```python
from build123d import *

# Parameters (mm, degrees)
F1_DEPTH = 3
F0_W     = 185
F0_H     = 265
F2_DEPTH = 74.8
F3_R     = 6.75
F4_R     = 2.99999


# Not quite as in the source:
# - a fillet or chamfer is up to 0.001 mm smaller than in the source, because OpenCascade refuses the exact size
# - ends of sketch curves that miss each other by under 0.0002 mm in the source are joined


with BuildPart() as f1:
    # F0 (on Top) → F1 (new body)
    with BuildSketch(Plane.XY):
        with BuildLine():
            Line((70.6, 125.95), (70.6, 129))
            Line((70.6, 129), (-70.6, 129))
            Line((-70.6, 129), (-70.6, 125.95))
            ThreePointArc((-70.6, 125.95), (-72.577029227, 121.177029227), (-77.35, 119.2))
            Line((-77.35, 119.2), (-89, 119.2))
            Line((-89, 119.2), (-89, 6.080118008))
            Line((-89, 6.080118008), (-86, 6.080118008))
            ThreePointArc((-86, 6.080118008), (-79.25, -0.669881992), (-86, -7.419881992))
            Line((-86, -7.419881992), (-89, -7.419881992))
            Line((-89, -7.419881992), (-89, -119.2))
            Line((-89, -119.2), (-77.3450501441, -119.2))
            ThreePointArc((-77.3450501441, -119.2), (-72.4815603684, -121.2692984284), (-70.6, -126.2084541623))
            Line((-70.6, -126.2084541623), (-70.6, -129))
            Line((-70.6, -129), (70.6, -129))
            Line((70.6, -129), (70.6, -125.95))
            ThreePointArc((70.6, -125.95), (72.577029227, -121.177029227), (77.35, -119.2))
            Line((77.35, -119.2), (89, -119.2))
            Line((89, -119.2), (89, -6.75))
            Line((89, -6.75), (86, -6.75))
            ThreePointArc((86, -6.75), (79.25, 0), (86, 6.75))
            Line((86, 6.75), (89, 6.75))
            Line((89, 6.75), (89, 119.2))
            Line((89, 119.2), (77.35, 119.2))
            ThreePointArc((77.35, 119.2), (72.577029227, 121.177029227), (70.6, 125.95))
        make_face()
    extrude(amount=F1_DEPTH)

    # F0 (on Top) → F2 (join)
    with BuildSketch(Plane.XY):
        Rectangle(F0_W, F0_H)
        Polygon((70.6, 129), (89, 129), (89, 119.2), (89, 6.75), (89, -6.75), (89, -119.2), (89, -129), (70.6, -129), (-70.6, -129), (-89, -129), (-89, -119.2), (-89, -7.419881992), (-89, 6.080118008), (-89, 119.2), (-89, 129), (-70.6, 129), align=None, mode=Mode.SUBTRACT)
        with BuildLine():
            Line((-77.3450501441, -119.2), (-89, -119.2))
            Line((-89, -119.2), (-89, -129))
            Line((-89, -129), (-70.6, -129))
            Line((-70.6, -129), (-70.6, -126.2084541623))
            ThreePointArc((-70.6, -126.2084541623), (-72.4815603684, -121.2692984284), (-77.3450501441, -119.2))
        make_face()
        with BuildLine():
            Line((89, -129), (89, -119.2))
            Line((89, -119.2), (77.35, -119.2))
            ThreePointArc((77.35, -119.2), (72.577029227, -121.177029227), (70.6, -125.95))
            Line((70.6, -125.95), (70.6, -129.000006485))
            Line((70.6, -129.000006485), (89, -129))
        make_face()
        with BuildLine():
            Line((-70.6, 125.95), (-70.6, 129))
            Line((-70.6, 129), (-89, 129))
            Line((-89, 129), (-89, 119.2))
            Line((-89, 119.2), (-77.35, 119.2))
            ThreePointArc((-77.35, 119.2), (-72.577029227, 121.177029227), (-70.6, 125.95))
        make_face()
        with BuildLine():
            Line((89, 119.2), (89, 129))
            Line((89, 129), (70.6, 129))
            Line((70.6, 129), (70.6, 125.95))
            ThreePointArc((70.6, 125.95), (72.577029227, 121.177029227), (77.35, 119.2))
            Line((77.35, 119.2), (89, 119.2))
        make_face()
        with BuildLine():
            Line((-86, 6.080118008), (-89, 6.080118008))
            Line((-89, 6.080118008), (-89, -7.419881992))
            Line((-89, -7.419881992), (-86, -7.419881992))
            ThreePointArc((-86, -7.419881992), (-79.25, -0.669881992), (-86, 6.080118008))
        make_face()
        with BuildLine():
            Line((89, -6.75), (89, 6.75))
            Line((89, 6.75), (86, 6.75))
            ThreePointArc((86, 6.75), (79.25, 0), (86, -6.75))
            Line((86, -6.75), (89, -6.75))
        make_face()
    extrude(amount=F2_DEPTH)

    # F3
    f3_edges = [f1.edges().sort_by_distance(p)[0] for p in [
        (-92.5, 132.5, 37.4),
        (92.5, 132.5, 37.4),
        (92.5, -132.5, 37.4),
        (-92.5, -132.5, 37.4),
    ]]
    fillet(f3_edges, radius=F3_R)

    # F4 (radius 3 in the source; OpenCascade refuses exactly that, so slightly less here)
    f4_edges = [f1.edges().sort_by_distance(p)[0] for p in [
        (-89, 6.080118, 38.9),
        (-89, 119.2, 38.9),
        (-70.6, 129, 38.9),
        (70.6, 129, 38.9),
        (89, 119.2, 38.9),
        (-89, -7.419882, 38.9),
        (89, 6.75, 38.9),
        (89, -6.75, 38.9),
        (-89, -119.2, 38.9),
        (-70.6, -129, 38.9),
        (70.6, -129, 38.9),
        (89, -119.2, 38.9),
    ]]
    fillet(f4_edges, radius=F4_R)


solid = f1.part
```
Build history of the part. All positions in model axes, mm. A direction names the side the tool comes from. Round coordinates to 2 decimals unless told otherwise and drop trailing zeros. Write each loop counter-clockwise with the first axis right and the second up, starting at its lowest first coordinate (ties: lowest second). Pieces come first, ordered by that corner, then holes. Notation, with made-up numbers: (-20.5, 12) - (16.5, 12) arc R22 ccw to (16.5, 31) - close; hole circle Ø5 at (48, 16). An arc over 180 degrees is marked (long way). Write each question's results on one line, items separated by ' | '. Start each with the question number.
Item 1: Which spindle directions (+Z, -Z, +X, -X, +Y, -Y) get a long thin tool onto all of the face, cutting with end or side? Do faces 1 (the face through (72.525, 121.23, 38.397)), 2 (the face through (-83, 1, 74.8)). Say none if no direction does.
Item 2: Saw through at B-B (x = 25). Write the cut outline in (y, z).
Item 3: Mould opens along Z. For faces 3 (the face through (92.5, -2, 37)), 4 (the face through (-1, 2, 0)), 5 (the face through (-1, 2, 3)) say: pulls with the +Z half, pulls with the -Z half, needs draft (parallel to the pull), parting line crosses it, or undercut.
Item 4: Wall check: L1, parallel to X at y = 47, z = 54; L2, parallel to Y at x = 67, z = 19; L3, parallel to Z at x = -45, y = 86. Give the ranges that are in metal, low to high. Write a range as [from, to].
Item 5: Saw through at A-A (y = 89). Write the cut outline in (x, z).
Results are:
1) face 1: +Z | face 2: +Z, +X, -X, +Y, -Y
2) outline: (-132.5, 0) - (132.5, 0) - (132.5, 74.8) - (129, 74.8) - (129, 3) - (-129, 3) - (-129, 74.8) - (-132.5, 74.8) - close
3) face 3: needs draft | face 4: pulls with the -Z half | face 5: pulls with the +Z half
4) L1: x = [-92.5, -89], [89, 92.5] | L2: y = [-132.5, -129], [129, 132.5] | L3: z = [0, 3]
5) outline: (-92.5, 0) - (92.5, 0) - (92.5, 74.8) - (89, 74.8) - (89, 3) - (-89, 3) - (-89, 74.8) - (-92.5, 74.8) - close
